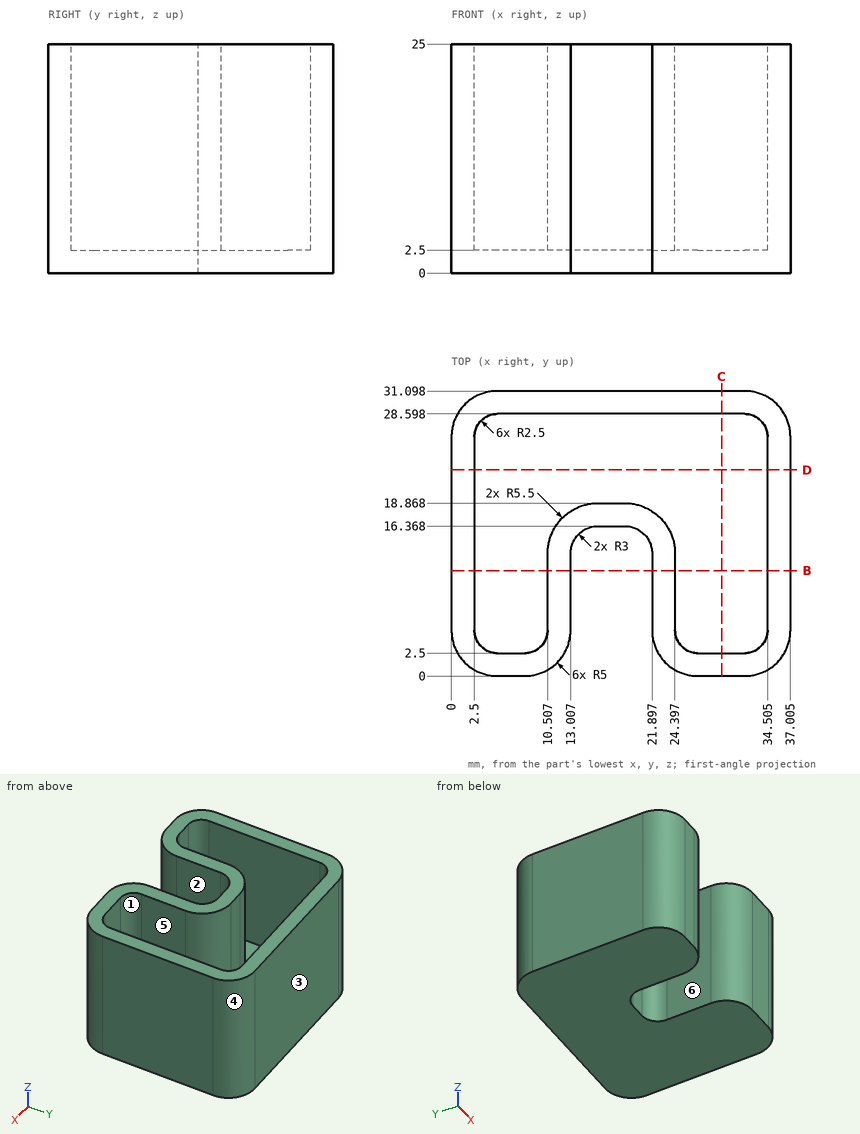
Input: dimensioned drawing with shaded views. Units: mm. Origin: part minimum x, y, z. A direction names the side the tool comes from. Coordinates: 2 decimals unless noted, no trailing zeros. Order: outer loops, then holes, each group sorted by start corner. A loop starts at its lowest first (then second) coordinate and runs counter-clockwise, first axis right, second up. Notation, with made-up numbers: (16.25, 55.5) - (63.25, 55.5) arc R25 ccw to (63.25, 91.5) - close; hole circle Ø7 at (31, -1.75). An arc over 180 degrees is marked (long way). One line per item, written item: value.
1) Ray query, line 1 (X direction, y = 13, z = 9.75) (1 decimal); line 2 (Y direction, x = 27.5, z = 21.25); line 3 (Y direction, x = 18.5, z = 13.5). Return the intervals inside material, ascending. Write a range as [from, to].
Computed values:
line 1: x = [0, 2.5], [10.5, 13], [21.9, 24.4], [34.5, 37]
line 2: y = [0, 2.5], [28.6, 31.1]
line 3: y = [16.37, 18.87], [28.6, 31.1]
2) Cut plane D-D on y = 22.5. Output: boundary loops of the cut face in (x, z) (1 decimal).
Computed values:
outline: (0, 0) - (37, 0) - (37, 25) - (34.5, 25) - (34.5, 2.5) - (2.5, 2.5) - (2.5, 25) - (0, 25) - close
3) Mould query, pull axis Y, two halves, no side actions, for the marked faces 4, 5 and 6. Classes: released by +Y, released by -Y, zero draft, split by the parting line, or undercut.
Computed values:
face 4: released by +Y
face 5: undercut
face 6: zero draft
4) Contact query for flat-ended pins moving along their axis: pin 1 (11 mm diameter, centred on x = 14, z = 17, fed in from -Y); pin 2 (3 mm diameter, centred on x = 23.5, y = 23.5, fed in from +Z); pin 3 (1 mm diameter, centred on y = 3.5, z = 9.5, fed in from -X). Output: stop coordinate, or through.
Computed values:
pin 1: stops at y = 0.02
pin 2: stops at z = 2.5
pin 3: stops at x = 0.1
5) Cut plane C-C on x = 29.5. Output: boundary loops of the cut face in (y, z), plus the area to 3 significant figures.
Computed values:
outline: (0, 0) - (31.1, 0) - (31.1, 25) - (28.6, 25) - (28.6, 2.5) - (2.5, 2.5) - (2.5, 25) - (0, 25) - close
area: 190 mm^2
6) Cut plane B-B on y = 11.5. Output: boundary loops of the cut face in (x, z) (1 decimal).
Computed values:
outline: (0, 0) - (13, 0) - (13, 25) - (10.5, 25) - (10.5, 2.5) - (2.5, 2.5) - (2.5, 25) - (0, 25) - close; (21.9, 0) - (37, 0) - (37, 25) - (34.5, 25) - (34.5, 2.5) - (24.4, 2.5) - (24.4, 25) - (21.9, 25) - close
7) Reachability of the marked faces 1, 2 and 3 from +Z, -Z, +X, -X, +Y, -Y: full face, straight path, thin tool, end or side. Return the list, or none.
Computed values:
face 1: +Z
face 2: +Z, -Z, -Y
face 3: +Z, -Z, +X, -X, +Y
